Source: CAD feature listing. Evaluate the final solid. Frame: model axes, mm. Give positions to 0.01 mm unless a question says otherwise; leave off trailing zeros. Write each loop counter-clockwise with the first axis right and the second up, starting at its lowest first coordinate (ties: lowest second). Pieces come first, ordered by that corner, then holes. Notation, with made-up numbers: M -34.75,55 L -17.75,55 A17 cw -17.75,62 Z; hole C 42,88.5 d9. An arc over 180 degrees is marked long. Answer as a JSON object with one key per item and string values. Group by question number.
```python
from build123d import *

# Parameters (mm, degrees)
SKETCH1_R           = 2.4
SKETCH1_R_2         = 1
BOSS_EXTRUDE1_DEPTH = 3.1


with BuildPart() as part:
    # Sketch1 → Boss-Extrude1 (new body)
    with BuildSketch(Plane.XY):
        with BuildLine():
            Line((-20.581998731, 60.620734864), (-17.522774409, 60.620734864))
            Line((-17.522774409, 60.620734864), (-13.723813298, 37.496124427))
            ThreePointArc((-13.723813298, 37.496124427), (-19.05238657, 31.220734864), (-24.380959842, 37.496124427))
            Line((-24.380959842, 37.496124427), (-20.581998731, 60.620734864))
        make_face()
        with Locations((-19.05238657, 36.620734864)):
            Circle(SKETCH1_R, mode=Mode.SUBTRACT)
        with Locations((-19.05238657, 57.620734864)):
            Circle(SKETCH1_R_2, mode=Mode.SUBTRACT)
    extrude(amount=BOSS_EXTRUDE1_DEPTH)


solid = part.part
```
(1) Ray query, L1, parallel to Y at x = -19.75, z = 1.35; L2, parallel to Y at x = -19.5, z = 0.85; L3, parallel to X at y = 57.25, z = 0.7. Return the intervals inside material, ascending. Write a range as [from, to].
(2) Pull-direction query (Y, two-part tool) for faces 1 (the flat face through (-19, 60.621, 2)), 2 (the flat face through (-19, 43, 3.1)), 3 (the cylindrical face through (-17.945, 34.492, 1.528)); classes: pulls with the +Y half, pulls with the -Y half, needs draft (parallel to the pull), parting line crosses it, or undercut.
(3) Section B-B, the plane z = 0.4. Return loops of the section in (x, y), plus the area to 3 significant figures.
(4) Section C-C, the plane y = 53. Return loops of the section in (x, z), plus the area to 3 significant figures.
(5) Contact query for a flat-ended pin moving along its axis: pin 1 Ø1.5 at (y, z) = (39.5, 1.5) entering from +X. Output: stop coordinate, or through.
(6) Section D-D, the plane x = -22.5. Return loops of the section in (y, z).
(7) Section A-A, the plane x = -19. Return loops of the section in (y, z).
Reported:
{
 "1": {"L1": "y = [31.27, 34.32], [38.92, 56.9], [58.34, 60.62]", "L2": "y = [31.24, 34.26], [38.98, 56.73], [58.51, 60.62]", "L3": "x = [-21.14, -19.98], [-18.12, -16.97]"},
 "2": {"face 1": "pulls with the +Y half", "face 2": "needs draft", "face 3": "undercut"},
 "3": {"outline": "M -24.38,37.5 A5.4 ccw long -13.72,37.5 L -17.52,60.62 L -20.58,60.62 Z; hole C -19.05,36.62 d4.8; hole C -19.05,57.62 d2", "area": "193 mm2"},
 "4": {"outline": "M -21.83,0 L -16.27,0 L -16.27,3.1 L -21.83,3.1 Z", "area": "17.2 mm2"},
 "5": {"pin 1": "stops at x = -13.93"},
 "6": {"outline": "M 32.46,0 L 48.95,0 L 48.95,3.1 L 32.46,3.1 Z"},
 "7": {"outline": "M 31.22,0 L 34.22,0 L 34.22,3.1 L 31.22,3.1 Z; M 39.02,0 L 56.62,0 L 56.62,3.1 L 39.02,3.1 Z; M 58.62,0 L 60.62,0 L 60.62,3.1 L 58.62,3.1 Z"}
}
